Job drawing, mm, ordinate dimensions from the low corner. One solid piece. Round coordinates to 2 decimals unless told otherwise and drop trailing zeros. Loops run counter-clockwise (first coordinate to the right, second up) from the corner with the lowest first, then second, coordinate; pieces in that order, holes last.
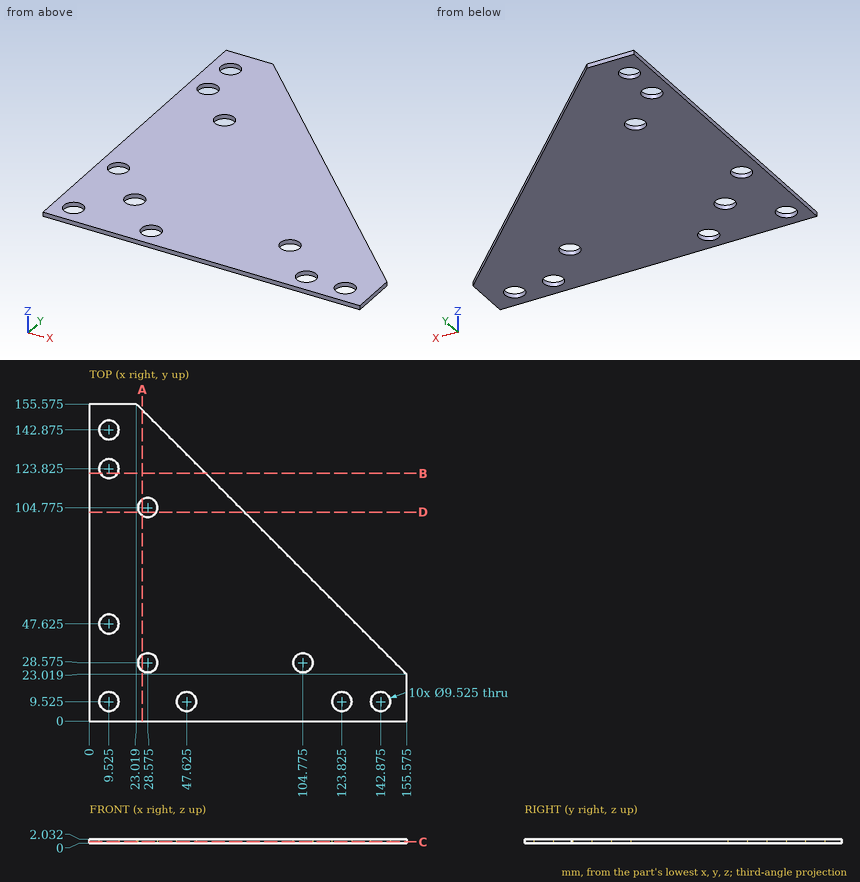
1) Slice it at B-B, the plane y = 121.5. Give the cut face in (x, z).
Values:
outline: (0, 0) - (5.37, 0) - (5.37, 2.03) - (0, 2.03) - close; (13.68, 0) - (57.09, 0) - (57.09, 2.03) - (13.68, 2.03) - close
2) Slice it at A-A, the plane x = 26. Give the cut face in (y, z).
Values:
outline: (0, 0) - (24.57, 0) - (24.57, 2.03) - (0, 2.03) - close; (32.58, 0) - (100.77, 0) - (100.77, 2.03) - (32.58, 2.03) - close; (108.78, 0) - (152.59, 0) - (152.59, 2.03) - (108.78, 2.03) - close
3) Slice it at D-D, the plane y = 102.5. Give the cut face in (x, z).
Values:
outline: (0, 0) - (24.39, 0) - (24.39, 2.03) - (0, 2.03) - close; (32.76, 0) - (76.09, 0) - (76.09, 2.03) - (32.76, 2.03) - close
4) Slice it at C-C, the plane z = 0.65. Give the number of separate pieces and of enclosed holes in the cut face, then the cut area to 3 significant figures.
Values:
separate pieces: 1
enclosed holes: 10
area: 14,700 mm2
5) Drop a flat-ended pin along its axis: pin 1 Ø1 at (x, z) = (122.5, 2) entering from -Y. Give the stop position or say it passes through.
Values:
pin 1: stops at y = 0
6) Wall check: line 1 along Y through (x, z) = (9.5, 0.3) (1 decimal); line 2 along X through (y, z) = (30.5, 1.95) (1 decimal); line 3 along X through (y, z) = (120.5, 1.7) (1 decimal). Give the ranges that are in metal, low to high.
Values:
line 1: y = 0 to 4.8, 14.3 to 42.9, 52.4 to 119.1, 128.6 to 138.1, 147.6 to 155.6
line 2: x = 0 to 24.2, 32.9 to 100.4, 109.1 to 148.1
line 3: x = 0 to 6.1, 12.9 to 58.1
